```python
from build123d import *

# Parameters (mm, degrees)
SKETCH1_R           = 2.5
BOSS_EXTRUDE1_DEPTH = 12
SKETCH3_R           = 0.25


with BuildPart() as part:
    # Sketch1 → Boss-Extrude1 (new body)
    with BuildSketch(Plane.XY):
        Circle(SKETCH1_R)
    extrude(amount=BOSS_EXTRUDE1_DEPTH)

    # Sweep1: sweep along a path in Sketch2
    with BuildLine(Plane(origin=(1, 0, 0), x_dir=(0, 0, -1), z_dir=(1, 0, 0))) as sweep1_path:
        Line((0, 0), (2, 0))
    # Sketch3 → Sweep1 (sweep)
    with BuildSketch(Plane(origin=(0, 0, 0), x_dir=(-1, 0, 0), z_dir=(0, 0, -1))):
        with Locations((-1, 0)):
            Circle(SKETCH3_R)
    sweep1 = sweep(path=sweep1_path.line)

    # Mirror1: Sweep1 across plane
    add(sweep1.mirror(Plane(origin=(0, 0, 0), x_dir=(0, 0, 1), z_dir=(1, 0, 0))))


solid = part.part
```
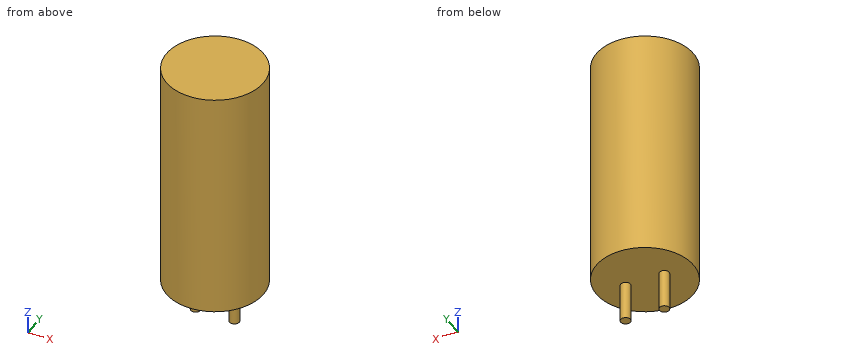
Could you check a few things on this model? Use its own coordinates, in mm. Round coordinates to 2 decimals unless told otherwise and drop trailing zeros. Write each loop counter-clockwise with the first axis right and the second up, starting at its lowest first coordinate (ties: lowest second). Pieces come first, ordered by that corner, then holes.
(1) Suppose I cut it at D-D on x = 0. Write out the boundary of the cut face in (y, z).
Findings below:
outline: (-2.5, 0) - (2.5, 0) - (2.5, 12) - (-2.5, 12) - close
(2) For pin 1 (2 mm diameter, centred on x = 0.5, y = 1.5, fed in from -Z); pin 2 (1 mm diameter, centred on x = 1, z = 4, fed in from -Y), each with a flat end and sliding along its axis, tell me the tip position at first contact or that it passes through.
Findings below:
pin 1: stops at z = 0
pin 2: stops at y = -2.45
(3) Suppose I cut it at B-B on x = 1. Write out the boundary of the cut face in (y, z).
Findings below:
outline: (-2.29, 0) - (-0.25, 0) - (-0.25, -2) - (0.25, -2) - (0.25, 0) - (2.29, 0) - (2.29, 12) - (-2.29, 12) - close
(4) Suppose I cut it at C-C on z = 10.75. Write out the boundary of the cut face in (x, y).
Findings below:
outline: circle Ø5 at (0, 0)
(5) If I drill on probe 1 along Z at (x, y) = (0.5, 2.2); probe 2 along X at (y, z) = (-0.1, 4.25); probe 3 along Y at (x, z) = (-0.8, 3.5), over which ranges is the centre line in solid material (lowest first)?
Findings below:
probe 1: z = 0 to 12
probe 2: x = -2.5 to 2.5
probe 3: y = -2.37 to 2.37
(6) Suppose I cut it at A-A on y = 0. Write out the boundary of the cut face in (x, z), and give its area (3 significant figures).
Findings below:
outline: (-2.5, 0) - (-1.25, 0) - (-1.25, -2) - (-0.75, -2) - (-0.75, 0) - (0.75, 0) - (0.75, -2) - (1.25, -2) - (1.25, 0) - (2.5, 0) - (2.5, 12) - (-2.5, 12) - close
area: 62.0 mm2
